Geometry check sheet. Reference: the model listing, model coordinates, mm. A direction names the side the tool comes from. Round coordinates to 2 decimals unless told otherwise and drop trailing zeros. Loops run counter-clockwise (first coordinate to the right, second up) from the corner with the lowest first, then second, coordinate; pieces in that order, holes last. Notation, with made-up numbers: M -8.75,70 L 24.25,70 A20 cw 24.25,103 Z; hole C 83,-34.75 d5. An arc over 180 degrees is marked long. Write item = value, one per line.
from build123d import *

# Parameters (mm, degrees)
SKETCH2_R           = 2
SKETCH2_W           = 5
SKETCH2_H           = 10
BOSS_EXTRUDE1_DEPTH = 6


with BuildPart() as part:
    # Sketch2 → Boss-Extrude1 (new body)
    with BuildSketch(Plane(origin=(0, 0, 0), x_dir=(1, 0, 0), z_dir=(0, 1, 0))):
        Polygon((-21.626106175, 30.870423783), (-11.626106175, 30.870423783), (-11.626106175, 27.870423783), (-1.626106175, 27.870423783), (-1.626106175, 30.870423783), (18.373893825, 30.870423783), (18.373893825, 27.870423783), (28.373893825, 27.870423783), (28.373893825, 30.870423783), (38.373893825, 30.870423783), (38.373893825, -19.129576217), (-21.626106175, -19.129576217), align=None)
        with Locations(Location((-13.626106175, 16.870423783, 0), (0, 0, 270))):
            Circle(SKETCH2_R, mode=Mode.SUBTRACT)
        with Locations(Location((-13.626106175, -5.129576217, 0), (0, 0, 270))):
            Circle(SKETCH2_R, mode=Mode.SUBTRACT)
        with Locations(Location((30.373893825, 16.870423783, 0), (0, 0, 270))):
            Circle(SKETCH2_R, mode=Mode.SUBTRACT)
        with Locations(Location((30.373893825, -5.129576217, 0), (0, 0, 270))):
            Circle(SKETCH2_R, mode=Mode.SUBTRACT)
        with Locations((20.873893825, 16.870423783)):
            Rectangle(SKETCH2_W, SKETCH2_H, mode=Mode.SUBTRACT)
        with Locations((-4.126106175, 16.870423783)):
            Rectangle(SKETCH2_W, SKETCH2_H, mode=Mode.SUBTRACT)
        with Locations((-4.126106175, -5.129576217)):
            Rectangle(SKETCH2_W, SKETCH2_H, mode=Mode.SUBTRACT)
        with Locations((20.873893825, -5.129576217)):
            Rectangle(SKETCH2_W, SKETCH2_H, mode=Mode.SUBTRACT)
    extrude(amount=BOSS_EXTRUDE1_DEPTH)


solid = part.part
(1) Sectioned sample at C-C on y = 1.6. State how many separate pieces and enclosed holes the cut face has, then the cut area to 3 significant figures.
Result set:
separate_pieces = 1
enclosed_holes = 8
area = 2,690 mm2
(2) Sectioned sample at A-A on x = 21. Record the cut outline in (y, z).
Result set:
outline = M 0,-27.87 L 6,-27.87 L 6,-21.87 L 0,-21.87 Z; M 0,-11.87 L 6,-11.87 L 6,0.13 L 0,0.13 Z; M 0,10.13 L 6,10.13 L 6,19.13 L 0,19.13 Z
(3) Tool access check on faces 1 (the flat face through (33, 3, -30.87)), 2 (the flat face through (-4, 3, -11.87)), 3 (the flat face through (-11.626, 3, -29)). Record the directions out of +Z, -Z, +X, -X, +Y, -Y that give a thin tool (end or side, any length) a straight path to the whole face; none if there is none.
Result set:
face_1 = -Z, +X, -X, +Y, -Y
face_2 = +Y, -Y
face_3 = -Z, +Y, -Y
(4) Release check for a two-part mould opening along X. For faces 4 (the flat face through (23, 3, -27.87)), 5 (the flat face through (9, 3, 19.13)), 6 (the flat face through (38.374, 3, -6)), 7 (the cylindrical face through (32.357, 2.958, -17.131)) record: released by +X, released by -X, zero draft, split by the parting line, or undercut.
Result set:
face_4 = undercut
face_5 = zero draft
face_6 = released by +X
face_7 = undercut
(5) Material ranges on line 1 along Z through (x, y) = (22, 1.55); line 2 along X through (y, z) = (4.85, 1.5); line 3 along X through (y, z) = (3.25, 4.5), recorded low to high. Write a range as from..to.
Result set:
line_1 = -27.87..-21.87, -11.87..0.13, 10.13..19.13
line_2 = -21.63..-6.63, -1.63..18.37, 23.37..38.37
line_3 = -21.63..-15.52, -11.73..-6.63, -1.63..18.37, 23.37..28.48, 32.27..38.37
(6) Sectioned sample at B-B on z = 8. Record the cut outline in (x, y).
Result set:
outline = M -21.63,0 L -6.63,0 L -6.63,6 L -21.63,6 Z; M -1.63,0 L 18.37,0 L 18.37,6 L -1.63,6 Z; M 23.37,0 L 38.37,0 L 38.37,6 L 23.37,6 Z
(7) Sectioned sample at D-D on z = -16. Record the cut outline in (x, y).
Result set:
outline = M -21.63,0 L -15.43,0 L -15.43,6 L -21.63,6 Z; M -11.83,0 L -6.63,0 L -6.63,6 L -11.83,6 Z; M -1.63,0 L 18.37,0 L 18.37,6 L -1.63,6 Z; M 23.37,0 L 28.57,0 L 28.57,6 L 23.37,6 Z; M 32.17,0 L 38.37,0 L 38.37,6 L 32.17,6 Z
